```python
from build123d import *

# Parameters (mm, degrees)
F1_DEPTH = 30.5
F2_R     = 2
F3_R     = 2


with BuildPart() as f1:
    # F0 (on Right) → F1 (new body)
    with BuildSketch(Plane.YZ):
        with BuildLine():
            Line((0, 6.9982859343), (0, 0))
            Line((0, 0), (50, 0))
            ThreePointArc((50, 0), (47.1879454394, 15.8045232241), (52.2596416003, 31.035035469))
            Line((52.2596416003, 31.035035469), (0, 6.9982859343))
        make_face()
    extrude(amount=F1_DEPTH)

    # F2
    f2_edges = [f1.edges().sort_by_distance(p)[0] for p in [
        (15.25, 52.259642, 31.035035),
    ]]
    fillet(f2_edges, radius=F2_R)

    # F3
    f3_edges = [f1.edges().sort_by_distance(p)[0] for p in [
        (15.25, 0, 6.998286),
        (15.25, 50, 0),
    ]]
    fillet(f3_edges, radius=F3_R)


solid = f1.part
```
Part model, mm, in its own coordinate system. Round coordinates to 2 decimals unless told otherwise and drop trailing zeros. Order: outer loops, then holes, each group sorted by start corner. A loop starts at its lowest first (then second) coordinate and runs counter-clockwise, first axis right, second up. Notation, with made-up numbers: M 50,48.5 L 57,48.5 A27 ccw 57,69.5 Z; hole C -27,38.25 d8. An arc over 180 degrees is marked long. Answer in a Markdown table with one row per item. Add a question column.
Q1. Pin check, flat tips, straight feed: pin 1 (5 mm diameter, centred on y = 31.5, z = 13, fed in from -X); pin 2 (10 mm diameter, centred on x = 26, z = 16, fed in from +Y); pin 3 (8 mm diameter, centred on x = 10.5, z = 12.5, fed in from +Y). Stop position of each tip, or through.
Q2. Cut at B-B on y = 40. Give the cut face in (x, z).
Q3. Wall check: L1, parallel to Z at x = 28.5, y = 44; L2, parallel to Y at x = 25, z = 15; L3, parallel to Z at x = 24.5, y = 20. Give the ranges that are in metal, low to high. Write a range as from..to.
Q4. Cut at C-C on z = 20.5. Give the cut face in (x, y), and give its area (3 significant figures).
Q5. Cut at A-A on x = 17. Give the cut face in (y, z).
Q6. Mould opens along Z. For faces 1 (the face through (15.036, 24.372, 18.208)), 2 (the face through (15.46, 48.69, 0.86)), 3 (the face through (30.5, 30, 11)) say: +Z half, -Z half, draft (parallel to the pull), parting line (faces both ways), or undercut.
Established:
| question | item | result |
|---|---|---|
| 1 | pin 1 | stops at x = 0 |
| 1 | pin 2 | stops at y = 47.99 |
| 1 | pin 3 | stops at y = 47.48 |
| 2 | outline | M 0,0 L 30.5,0 L 30.5,25.4 L 0,25.4 Z |
| 3 | L1 | z = 0..27.24 |
| 3 | L2 | y = 17.4..47.14 |
| 3 | L3 | z = 0..16.2 |
| 4 | outline | M 0,29.35 L 30.5,29.35 L 30.5,47.88 L 0,47.88 Z |
| 4 | area | 565 mm2 |
| 5 | outline | M 0,0 L 47.05,0 A2 ccw 48.93,2.66 A32.6 cw 49.62,26 A2 ccw 46.94,28.59 L 1.16,7.53 A2 ccw 0,5.72 Z |
| 6 | face 1 | +Z half |
| 6 | face 2 | undercut |
| 6 | face 3 | draft |
